```python
from build123d import *

# Parameters (mm, degrees)
SKETCH_R   = 210
SKETCH_R_2 = 32
SKETCH_R_3 = 2.5
SKETCH_W   = 22
SKETCH_H   = 100
SKETCH_W_2 = 110
SKETCH_H_2 = 70
PAD_DEPTH  = 1.5


with BuildPart() as part:
    # Sketch → Pad (new body, symmetric)
    with BuildSketch(Plane.XY):
        Circle(SKETCH_R)
        with Locations((0, 170)):
            Circle(SKETCH_R_2, mode=Mode.SUBTRACT)
        with Locations((0, -170)):
            Circle(SKETCH_R_2, mode=Mode.SUBTRACT)
        with Locations((-141, 33.5)):
            Circle(SKETCH_R_3, mode=Mode.SUBTRACT)
        with Locations((-141, -33.5)):
            Circle(SKETCH_R_3, mode=Mode.SUBTRACT)
        with Locations((-115, 33.5)):
            Circle(SKETCH_R_3, mode=Mode.SUBTRACT)
        with Locations((-115, -33.5)):
            Circle(SKETCH_R_3, mode=Mode.SUBTRACT)
        with Locations((115, 33.5)):
            Circle(SKETCH_R_3, mode=Mode.SUBTRACT)
        with Locations((115, -33.5)):
            Circle(SKETCH_R_3, mode=Mode.SUBTRACT)
        with Locations((145, 33.5)):
            Circle(SKETCH_R_3, mode=Mode.SUBTRACT)
        with Locations((145, -33.5)):
            Circle(SKETCH_R_3, mode=Mode.SUBTRACT)
        with Locations((-90, 172.29129)):
            Circle(SKETCH_R_3, mode=Mode.SUBTRACT)
        with Locations((90, 172.29129)):
            Circle(SKETCH_R_3, mode=Mode.SUBTRACT)
        with Locations((-30, 200)):
            Circle(SKETCH_R_3, mode=Mode.SUBTRACT)
        with Locations((30, 200)):
            Circle(SKETCH_R_3, mode=Mode.SUBTRACT)
        with Locations((-30, 140)):
            Circle(SKETCH_R_3, mode=Mode.SUBTRACT)
        with Locations((30, 140)):
            Circle(SKETCH_R_3, mode=Mode.SUBTRACT)
        with Locations((-30, -140)):
            Circle(SKETCH_R_3, mode=Mode.SUBTRACT)
        with Locations((30, -140)):
            Circle(SKETCH_R_3, mode=Mode.SUBTRACT)
        with Locations((-30, -200)):
            Circle(SKETCH_R_3, mode=Mode.SUBTRACT)
        with Locations((30, -200)):
            Circle(SKETCH_R_3, mode=Mode.SUBTRACT)
        with Locations((-172, 0)):
            Rectangle(SKETCH_W, SKETCH_H, mode=Mode.SUBTRACT)
        with Locations((172, 0)):
            Rectangle(SKETCH_W, SKETCH_H, mode=Mode.SUBTRACT)
        with Locations((0, 90)):
            Rectangle(SKETCH_W_2, SKETCH_H_2, mode=Mode.SUBTRACT)
    extrude(amount=PAD_DEPTH, both=True)


solid = part.part
```
Design review of the part built by this model. Coordinates are the model's own, in mm. Give positions to 0.01 mm unless a question says otherwise; leave off trailing zeros. Order: outer loops, then holes, each group sorted by start corner. A loop starts at its lowest first (then second) coordinate and runs counter-clockwise, first axis right, second up. Notation, with made-up numbers: (18.5, 25.25) - (48.5, 25.25) arc R20 cw to (48.5, 40.25) - close; hole circle Ø6 at (58, 17). An arc over 180 degrees is marked (long way). Use a Markdown table: item, result. Add a question column.
(1) Add section D-D on x = -71.5. Give the boundary of the cut face in (y, z).
(2) Wall thickness on probe 1 along X at (y, z) = (-4, -1.25); probe 2 along Y at (x, z) = (-115, -0.8); probe 3 along Y at (x, z) = (9, 0.65): over which ranges is each line inside the solid? List them lowest first. Write a range as [from, to].
(3) Add section B-B on y = -44.5. Give the boundary of the cut face in (x, z), then the cut area to 3 significant figures.
(4) Mouldability with a two-part tool opening along X and no side actions: class faces 1 (the face through (200.3, 63.08, 0.02)), 2 (the face through (-4.166, -138.272, -0.021)), 3 (the face through (-3, 3, -1.5)), 4 (the face through (-4.166, 201.728, -0.021)) as +X half, -X half, draft (parallel to the pull), parting line (faces both ways), or undercut.
(5) Clearance check with flat-ended pins moving along their axes: P1, Ø1.5, axis at x = -125, z = 1, coming from the -Y side; P2, Ø0.9, axis at y = -12, z = 0.5, coming from the +X side; P3, Ø0.9, axis at y = 75, z = 0, coming from the +X side. State where each tip first meets the part, or that it passes through.
(6) Add section A-A on x = 0. Give the boundary of the cut face in (y, z), then the cut area to 3 significant figures.
(7) Add section C-C on z = -0.9. Give the number of separate pieces and of enclosed holes in the cut face, then the cut area to 3 significant figures.
Report:
| question | item | result |
|---|---|---|
| 1 | outline | (-197.45, -1.5) - (197.45, -1.5) - (197.45, 1.5) - (-197.45, 1.5) - close |
| 2 | probe 1 | x = [-209.96, -183], [-161, 161], [183, 209.96] |
| 2 | probe 2 | y = [-175.71, -36], [-31, 31], [36, 175.71] |
| 2 | probe 3 | y = [-209.81, -200.71], [-139.29, 55], [125, 139.29], [200.71, 209.81] |
| 3 | outline | (-205.23, -1.5) - (-183, -1.5) - (-183, 1.5) - (-205.23, 1.5) - close; (-161, -1.5) - (161, -1.5) - (161, 1.5) - (-161, 1.5) - close; (183, -1.5) - (205.23, -1.5) - (205.23, 1.5) - (183, 1.5) - close |
| 3 | area | 1,100 mm² |
| 4 | face 1 | parting line |
| 4 | face 2 | undercut |
| 4 | face 3 | draft |
| 4 | face 4 | undercut |
| 5 | P1 | stops at y = -169.3 |
| 5 | P2 | stops at x = 209.68 |
| 5 | P3 | stops at x = 196.32 |
| 6 | outline | (-210, -1.5) - (-202, -1.5) - (-202, 1.5) - (-210, 1.5) - close; (-138, -1.5) - (55, -1.5) - (55, 1.5) - (-138, 1.5) - close; (125, -1.5) - (138, -1.5) - (138, 1.5) - (125, 1.5) - close; (202, -1.5) - (210, -1.5) - (210, 1.5) - (202, 1.5) - close |
| 6 | area | 666 mm² |
| 7 | separate pieces | 1 |
| 7 | enclosed holes | 23 |
| 7 | area | 120,000 mm² |
